Autodesk Inventor part; units mm, degrees
ref_plane "YZ Plane" through (0, 0, 0) normal (1, 0, 0) x (0, 1, 0)
ref_plane "XZ Plane" through (0, 0, 0) normal (0, 1, 0) x (-1, 0, 0)
ref_plane "XY Plane" through (0, 0, 0) normal (0, 0, 1) x (1, 0, 0)
sketch "Boceto1" plane through (0, 0, 0) normal (0, 1, 0) x (-1, 0, 0)
  circle A0 centre (0, 0) radius 4.5
  dimension "d0" = 9
extrude "Extrusión1" add sketch "Boceto1" along normal blind 1.6
sketch "Boceto2" plane through (0, 1.6, 0) normal (0, 1, 0) x (1, 0, 0)
  circle A0 centre (0, 0) radius 2.5
  dimension "d3" = 5
extrude "Extrusión2" add sketch "Boceto2" along normal blind 55
fillet "Empalme1" radius 0.4 1 edges at (4.5, 0, 0)
fillet "Empalme2" radius 0.2 1 edges at (4.5, 1.6, 0)
sketch "Boceto3" plane through (0, 0, 0) normal (0, -1, 0) x (1, 0, 0)
  line L0 (-1.7321, 0) -> (-0.866, 1.5)
  line L1 (-0.866, 1.5) -> (0.866, 1.5)
  line L2 (0.866, 1.5) -> (1.7321, 0)
  line L3 (1.7321, 0) -> (0.866, -1.5)
  line L4 (0.866, -1.5) -> (-0.866, -1.5)
  line L5 (-0.866, -1.5) -> (-1.7321, 0)
  point P0 (0, 0)
  point P1 (0, 0)
  dimension "d8" = 3
extrude "Extrusión3" cut sketch "Boceto3" against normal blind 2.5
chamfer "Chaflán1" distance 0.5 angle 45 1 edges at (-2.5, 56.6, 0)
thread "Rosca2"
properties part number "m5x55" material "Hierro, gris"
Check sheet for the modelled part. Datum: model origin and axes. Units: mm. A direction names the side the tool comes from. Round coordinates to 2 decimals unless told otherwise and drop trailing zeros. Write each loop counter-clockwise with the first axis right and the second up, starting at its lowest first coordinate (ties: lowest second). Pieces come first, ordered by that corner, then holes. Notation, with made-up numbers: M 5.5,84 L 40.5,84 A23 ccw 40.5,110 Z; hole C 63,11.25 d3. An arc over 180 degrees is marked long. Write item = value, one per line. Start each with the question number.
1. Section check B-B, the plane y = 41. Record the cut outline in (x, z), then the cut area to 3 significant figures.
2. Tool access check on faces 4 (the flat face through (1.305, 1.232, -0.74)), 5 (the flat face through (0, 56.6, 0)), 6 (the cylindrical face through (-0.54, 28.47, -2.44)). Record the directions out of +Z, -Z, +X, -X, +Y, -Y that give a thin tool (end or side, any length) a straight path to the whole face; none if there is none.
3. Release check for a two-part mould opening along Z. For faces 1 (the flat face through (0, 1, 1.5)), 2 (the flat face through (-2, 1.6, -2)), 3 (the cylindrical face through (0.59, 0.89, -4.46)) record: pulls with the +Z half, pulls with the -Z half, needs draft (parallel to the pull), parting line crosses it, or undercut.
4. Section check A-A, the plane x = 0. Record the cut outline in (y, z), then the cut area to 3 significant figures.
5. Scan lines: line 1 (X direction, y = 51.5, z = 1.5); line 2 (Y direction, x = -2.75, z = 2); line 3 (Y direction, x = 0, z = 0.5). Record each from-to range of solid material in increasing order. Write a range as [from, to].
6. Gauge pin test, flat ends, axial feed: pin 1 (3 mm diameter, centred on x = 1, y = 8, fed in from -Z); pin 2 (5 mm diameter, centred on y = 10.5, z = -2, fed in from +X); pin 3 (5 mm diameter, centred on x = 0.5, y = 6, fed in from +Z). Record the tip position at first contact, or that the pin passes through.
Results found:
q1.outline = C 0,0 d5
q1.area = 19.6 mm^2
q2.face_4 = -Y
q2.face_5 = +Z, -Z, +X, -X, +Y
q2.face_6 = +Y
q3.face_1 = undercut
q3.face_2 = needs draft
q3.face_3 = parting line crosses it
q4.outline = M 0,-4.1 A0.4 ccw 0.4,-4.5 L 1.4,-4.5 A0.2 ccw 1.6,-4.3 L 1.6,-2.5 L 56.1,-2.5 L 56.6,-2 L 56.6,2 L 56.1,2.5 L 1.6,2.5 L 1.6,4.3 A0.2 ccw 1.4,4.5 L 0.4,4.5 A0.4 ccw 0,4.1 L 0,1.5 L 2.5,1.5 L 2.5,-1.5 L 0,-1.5 Z
q4.area = 282 mm^2
q5.line_1 = [-2, 2]
q5.line_2 = [0, 1.6]
q5.line_3 = [2.5, 56.6]
q6.pin_1 = -2.5
q6.pin_2 = 2.5
q6.pin_3 = 2.5
